Check sheet for the modelled part. Datum: model origin and axes. Units: mm. A direction names the side the tool comes from. Give positions to 0.01 mm unless a question says otherwise; leave off trailing zeros. Write each loop counter-clockwise with the first axis right and the second up, starting at its lowest first coordinate (ties: lowest second). Pieces come first, ordered by that corner, then holes. Notation, with made-up numbers: M -16,45.5 L 26,45.5 A16 ccw 26,76.5 Z; hole C -13.5,56 d7. An arc over 180 degrees is marked long. Write item = value, one per line. Start each with the question number.
1) Cross-section at D-D, the plane x = -17. Record the cut outline in (y, z), plus the area to 3 significant figures.
2) Go/stop test with flat-tipped pins: pin 1 (14 mm diameter, centred on y = -37, z = 3, fed in from +X); pin 2 (10 mm diameter, centred on x = 14.5, y = -41, fed in from -Z); pin 3 (3 mm diameter, centred on x = 13.5, y = -50.5, fed in from +Z). Record where each tip stops, or that it passes through.
3) Access from +Z, -Z, +X, -X, +Y, -Y to the whole of each face (thin tool, end or side, straight path). Record for faces 5 (the flat face through (17.539, -44, 6)), 6 (the flat face through (-15, -49.201, 8)), 7 (the flat face through (-15, -18.251, 2)), 8 (the flat face through (-17.52, -12.52, 27.84)), 9 (the flat face through (-15, -64, 12.7)).
4) Mould release check, pull along Y, two halves, no side actions. Record for faces 1 (the flat face through (-15, -45, 3.048)), 2 (the flat face through (2, -25.4, 25)), 3 (the flat face through (-45.961, -44, 6)), 4 (the flat face through (-7, 0, 18)): released by +Y, released by -Y, zero draft, split by the parting line, or undercut.
5) Cross-section at A-A, the plane z = 11.5. Record the cut outline in (x, y).
6) Cross-section at B-B, the plane x = 8. Record the cut outline in (y, z).
7) Cross-section at C-C, the plane y = -68. Record the cut outline in (x, z).
8) Scan lines: line 1 along Y through (x, z) = (-20, 10); line 2 along Y through (x, z) = (25.5, 42); line 3 along Y through (x, z) = (-40, 6.5). Record each from-to range of solid material in increasing order. Write a range as [from, to].
```python
from build123d import *

# Parameters (mm, degrees)
F0_W     = 63.5
F0_H     = 12.7
F1_DEPTH = 25.4
F2_W     = 63.5
F2_H     = 12.7
F3_DEPTH = 63.5
F4_W     = 63.5
F4_H     = 53.356215
F5_DEPTH = 3.048
F7_DEPTH = 25.4


with BuildPart() as f1:
    # F0 (on Front) → F1 (new body)
    with BuildSketch(Plane.XZ):
        with Locations((-14.211346, 6.35)):
            Rectangle(F0_W, F0_H)
        with BuildLine():
            Line((10.138772, 42.563359), (-45.961346, 12.7))
            Line((-45.961346, 12.7), (17.538654, 12.7))
            Line((17.538654, 12.7), (17.485546, 12.914324))
            ThreePointArc((17.485546, 12.914324), (2.252939, 24.874567), (10.138772, 42.563359))
        make_face()
        with BuildLine():
            Line((12.158692, 34.41166), (10.138772, 42.563359))
            ThreePointArc((10.138772, 42.563359), (2.252939, 24.874567), (17.485546, 12.914324))
            Line((17.485546, 12.914324), (15.465626, 21.066023))
            ThreePointArc((15.465626, 21.066023), (9.895796, 26.768401), (12.158692, 34.41166))
        make_face()
        with BuildLine():
            ThreePointArc((33.286654, 28.662235), (25.646248, 42.162843), (10.138772, 42.563359))
            Line((10.138772, 42.563359), (12.158692, 34.41166))
            ThreePointArc((12.158692, 34.41166), (20.672187, 35.885866), (25.412654, 28.662235))
            ThreePointArc((25.412654, 28.662235), (22.31761, 22.404324), (15.465626, 21.066023))
            Line((15.465626, 21.066023), (17.485546, 12.914324))
            ThreePointArc((17.485546, 12.914324), (28.655379, 17.507956), (33.286654, 28.662235))
        make_face()
    extrude(amount=F1_DEPTH)

    # F2 (on face) → F3 (join)
    with BuildSketch(Plane.XZ.offset(25.4)):
        with Locations((-14.211346, 6.35)):
            Rectangle(F2_W, F2_H)
    extrude(amount=F3_DEPTH)

    # F4 (on face) → F5 (cut)
    with BuildSketch(Plane(origin=(0, 0, 0), x_dir=(1, 0, 0), z_dir=(0, 0, -1))):
        with Locations((-14.211346, 44.929125)):
            Rectangle(F4_W, F4_H)
    extrude(amount=-F5_DEPTH, mode=Mode.SUBTRACT)

    # F6 (on face) → F7 (cut)
    with BuildSketch(Plane.XY.offset(12.7)):
        with BuildLine():
            ThreePointArc((-34.139643, -49.201058), (-30.283279, -51.341679), (-28.751483, -55.47779))
            ThreePointArc((-28.751483, -55.47779), (-30.551195, -59.906941), (-34.930185, -61.825479))
            Line((-34.930185, -61.825479), (4.326623, -61.822998))
            ThreePointArc((4.326623, -61.822998), (-2.004218, -55.971033), (3.333617, -49.201058))
            Line((3.333617, -49.201058), (-34.139643, -49.201058))
        make_face()
        with BuildLine():
            ThreePointArc((-34.930185, -61.825479), (-30.551195, -59.906941), (-28.751483, -55.47779))
            ThreePointArc((-28.751483, -55.47779), (-30.283279, -51.341679), (-34.139643, -49.201058))
            ThreePointArc((-34.139643, -49.201058), (-41.426093, -54.910512), (-35.271977, -61.8255))
            Line((-35.271977, -61.8255), (-34.930185, -61.825479))
        make_face()
        with BuildLine():
            ThreePointArc((10.676221, -55.472998), (8.450507, -50.644668), (3.333617, -49.201058))
            ThreePointArc((3.333617, -49.201058), (-2.004218, -55.971033), (4.326623, -61.822998))
            ThreePointArc((4.326623, -61.822998), (8.816491, -59.962984), (10.676221, -55.472998))
        make_face()
    extrude(amount=-F7_DEPTH, mode=Mode.SUBTRACT)


solid = f1.part
```
Reply:
q1.outline = M -88.9,0 L -71.61,0 L -71.61,3.05 L -61.82,3.05 L -61.82,12.7 L -88.9,12.7 Z; M -49.2,3.05 L -18.25,3.05 L -18.25,0 L 0,0 L 0,28.12 L -25.4,28.12 L -25.4,12.7 L -49.2,12.7 Z
q1.area = 1,240 mm2
q2.pin_1 = 17.54
q2.pin_2 = 3.05
q2.pin_3 = 12.7
q3.face_5 = -Z, +X, +Y, -Y
q3.face_6 = +Z, -Z
q3.face_7 = -Z, +X, -X
q3.face_8 = +Z, -X, +Y, -Y
q3.face_9 = +Z, +X, -X, -Y
q4.face_1 = undercut
q4.face_2 = released by -Y
q4.face_3 = zero draft
q4.face_4 = released by +Y
q5.outline = M -45.96,-88.9 L 17.54,-88.9 L 17.54,0 L -45.96,0 Z; hole M -35.27,-61.83 L -34.93,-61.83 L 4.33,-61.82 A6.35 ccw 10.68,-55.47 A6.35 ccw 3.33,-49.2 L -34.14,-49.2 A6.35 ccw long Z
q6.outline = M -88.9,0 L -71.61,0 L -71.61,3.05 L -60.65,3.05 L -60.65,12.7 L -88.9,12.7 Z; M -50.29,3.05 L -18.25,3.05 L -18.25,0 L 0,0 L 0,41.42 L -25.4,41.42 L -25.4,12.7 L -50.29,12.7 Z
q7.outline = M -45.96,3.05 L 17.54,3.05 L 17.54,12.7 L -45.96,12.7 Z
q8.line_1 = [-88.9, -61.82], [-49.2, 0]
q8.line_2 = [-25.4, 0]
q8.line_3 = [-88.9, -59.52], [-51.44, 0]
